Part print with two shaded views. Sizes in mm from the minimum x, y, z corner. Coordinates: 2 decimals unless noted, no trailing zeros. Loops run counter-clockwise (first coordinate to the right, second up) from the corner with the lowest first, then second, coordinate; pieces in that order, holes last. Notation, with made-up numbers: (37.25, 26.25) - (47.25, 26.25) arc R14 ccw to (47.25, 48.25) - close; hole circle Ø8 at (-12, 25). An arc over 180 degrees is marked (long way). Answer as CSV lines item,"result".
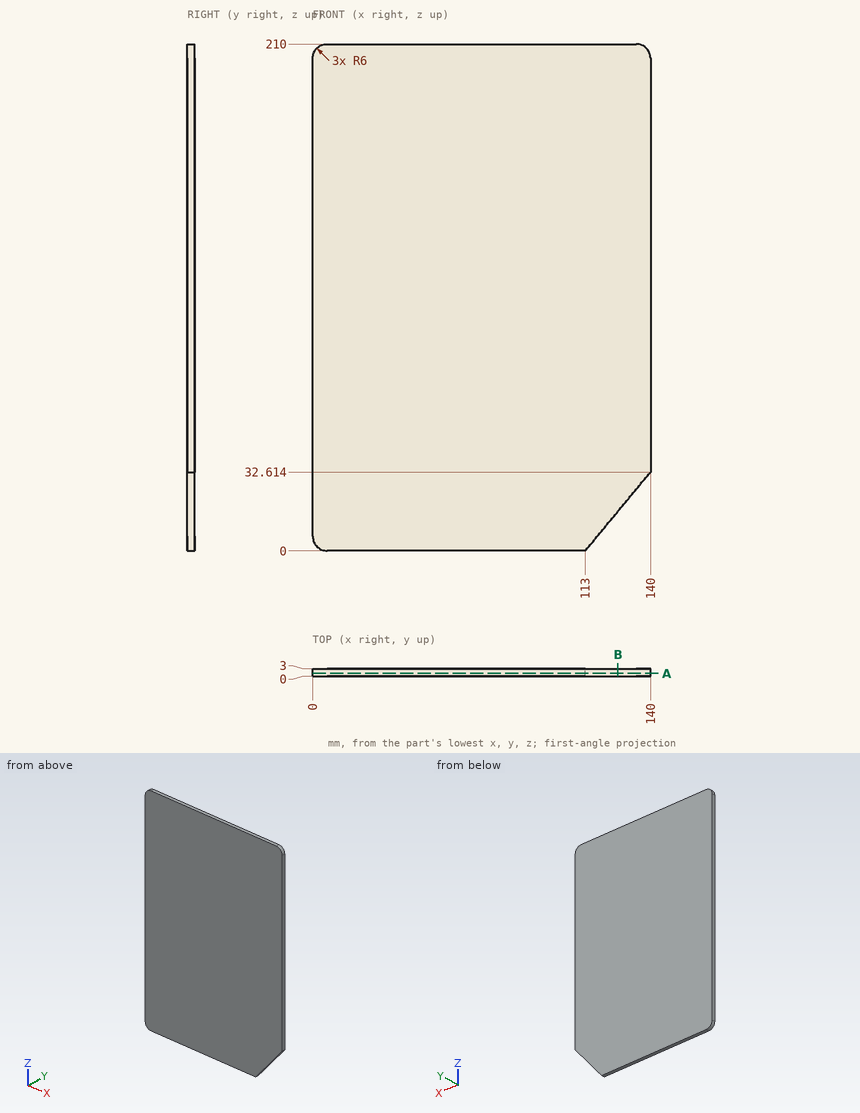
Q1. Saw through at B-B (x = 126.5). Give the cut face in (y, z), then the cut area to 3 significant figures.
Results:
outline,"(0, 16.31) - (3, 16.31) - (3, 210) - (0, 210) - close"
area,"581 mm^2"
Q2. Saw through at A-A (y = 1.1). Give the cut face in (x, z), then the cut area to 3 significant figures.
Results:
outline,"(0, 6) arc R6 ccw to (6, 0) - (113, 0) - (140, 32.61) - (140, 204) arc R6 ccw to (134, 210) - (6, 210) arc R6 ccw to (0, 204) - close"
area,"28,900 mm^2"
Q3. Wall check: L1, parallel to Z at x = 118, y = 2.5; L2, parallel to Z at x = 132.5, y = 1.1 (1 decimal). Give the ranges that are in metal, low to high.
Results:
L1,"z = 6.04 to 210"
L2,"z = 23.6 to 210"
